For this review, take the finished solid that the model builds, in its own axes (mm). Face numbers are marked on the shaded views. A direction names the side the tool comes from. Round coordinates to 2 decimals unless told otherwise and drop trailing zeros. Loops run counter-clockwise (first coordinate to the right, second up) from the corner with the lowest first, then second, coordinate; pieces in that order, holes last. Notation, with made-up numbers: (80.25, 42.25) -> (105.25, 42.25) arc R23 ccw to (105.25, 69.25) -> close; hole circle Ø2 at (47, -37.5). An arc over 180 degrees is marked (long way). One line per question, with ' | ' between items. Start each with the question number.
1. Consider section D-D (y = -4.75). Write out the cut boundary in (x, z).
2. For pin 1 Ø1 at (x, z) = (-6, 8) entering from +Y; pin 2 Ø3 at (x, z) = (-9.5, 1.5) entering from +Y; pin 3 Ø1 at (y, z) = (1.5, -4.5) entering from +X, all flat-tipped, find the tip position at first contact; note any pin that passes through.
3. Consider section C-C (y = -1.25). Write out the cut boundary in (x, z) (3 decimals), and give its area (3 significant figures).
4. Consider section B-B (z = 16.25). Write out the cut boundary in (x, y).
5. Draft analysis for pull direction X (two halves, no side actions). For the marked faces 4, 5, 6 and 7, state which applies: pulls with the +X half, pulls with the -X half, needs draft (parallel to the pull), parting line crosses it, or undercut.
6. Consider section A-A (x = -9). Write out the cut boundary in (y, z), and give its area (3 significant figures).
7. For the marked faces 1, 2 and 3, list the 3-axis set-ups (+Z, -Z, +X, -X, +Y, -Y) from which the entire face can be reached by the end or side of a thin tool; tool diameter is ignored.
8. Wall thickness on line 1 along Z through (x, y) = (5, -4.75); line 2 along Z through (x, y) = (-9, 0.25); line 3 along Y through (x, z) = (5.75, -17.5): over which ranges is each line inside the solid? List them lowest first.
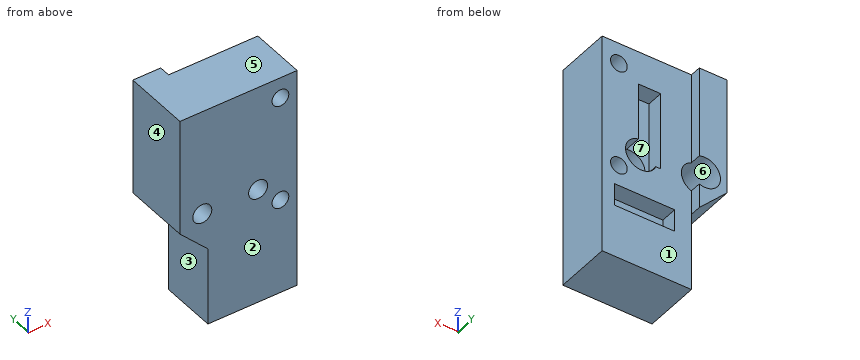
```python
from build123d import *

# Parameters (mm, degrees)
BOX025_W               = 20
BOX025_H               = 10
BOX025_DEPTH           = 44
BOX027_W               = 10.75
BOX027_H               = 10
BOX027_DEPTH           = 4
BOX026_W               = 4
BOX026_H               = 10
BOX026_DEPTH           = 14
CYLINDER031_R          = 2.8
CYLINDER031_DEPTH      = 22
CYLINDER031_ROLL_ANGLE = 90
CYLINDER027_R          = 1.5
CYLINDER027_DEPTH      = 22
CYLINDER027_ROLL_ANGLE = 90
CYLINDER029_R          = 1.5
CYLINDER029_DEPTH      = 22
CYLINDER029_ROLL_ANGLE = 90
CYLINDER026_R          = 1.7
CYLINDER026_DEPTH      = 22
CYLINDER026_ROLL_ANGLE = 90
CYLINDER028_R          = 1.7
CYLINDER028_DEPTH      = 22
CYLINDER028_ROLL_ANGLE = 90
CYLINDER030_R          = 2.8
CYLINDER030_DEPTH      = 22
CYLINDER030_ROLL_ANGLE = 90
PAD016_DEPTH           = 12


with BuildPart() as cube025:
    # Box025 → Box025 (new body)
    with BuildSketch(Plane(origin=(-8, 0, -22), x_dir=(1, 0, 0), z_dir=(0, 0, 1))):
        with Locations((10, 5)):
            Rectangle(BOX025_W, BOX025_H)
    extrude(amount=BOX025_DEPTH)


with BuildPart() as cube027:
    # Box027 → Box027 (new body)
    with BuildSketch(Plane(origin=(-5, -3, -10.5), x_dir=(1, 0, 0), z_dir=(0, 0, 1))):
        with Locations((5.375, 5)):
            Rectangle(BOX027_W, BOX027_H)
    extrude(amount=BOX027_DEPTH)


with BuildPart() as fusion025:
    # Box026 → Box026 (new body)
    with BuildSketch(Plane(origin=(-2.5, -3, 0), x_dir=(1, 0, 0), z_dir=(0, 0, 1))):
        with Locations((2, 5)):
            Rectangle(BOX026_W, BOX026_H)
    extrude(amount=BOX026_DEPTH)

    # Fusion025: union Cube027
    add(cube027.part)


with BuildPart() as cylinder031:
    # Cylinder031 → Cylinder031 (new body)
    with BuildSketch(Plane.XY):
        Circle(CYLINDER031_R)
    extrude(amount=CYLINDER031_DEPTH)


with BuildPart() as cylinder031_1:
    # Cylinder031 roll: moved
    add(cylinder031.part.rotate(Axis((0, 0, 0), (1, 0, 0)), CYLINDER031_ROLL_ANGLE))


with BuildPart() as cylinder031_2:
    # Cylinder031 placement: moved
    add(cylinder031_1.part.moved(Location((-9, 15, 1))))


with BuildPart() as cylinder027:
    # Cylinder027 → Cylinder027 (new body)
    with BuildSketch(Plane.XY):
        Circle(CYLINDER027_R)
    extrude(amount=CYLINDER027_DEPTH)


with BuildPart() as cylinder027_1:
    # Cylinder027 roll: moved
    add(cylinder027.part.rotate(Axis((0, 0, 0), (1, 0, 0)), CYLINDER027_ROLL_ANGLE))


with BuildPart() as cylinder027_2:
    # Cylinder027 placement: moved
    add(cylinder027_1.part.moved(Location((5, 6, 16.25))))


with BuildPart() as cylinder029:
    # Cylinder029 → Cylinder029 (new body)
    with BuildSketch(Plane.XY):
        Circle(CYLINDER029_R)
    extrude(amount=CYLINDER029_DEPTH)


with BuildPart() as cylinder029_1:
    # Cylinder029 roll: moved
    add(cylinder029.part.rotate(Axis((0, 0, 0), (1, 0, 0)), CYLINDER029_ROLL_ANGLE))


with BuildPart() as cylinder029_2:
    # Cylinder029 placement: moved
    add(cylinder029_1.part.moved(Location((5, 6, -2.75))))


with BuildPart() as cylinder026:
    # Cylinder026 → Cylinder026 (new body)
    with BuildSketch(Plane.XY):
        Circle(CYLINDER026_R)
    extrude(amount=CYLINDER026_DEPTH)


with BuildPart() as cylinder026_1:
    # Cylinder026 roll: moved
    add(cylinder026.part.rotate(Axis((0, 0, 0), (1, 0, 0)), CYLINDER026_ROLL_ANGLE))


with BuildPart() as cylinder026_2:
    # Cylinder026 placement: moved
    add(cylinder026_1.part.moved(Location((-9, 6, 1))))


with BuildPart() as cylinder028:
    # Cylinder028 → Cylinder028 (new body)
    with BuildSketch(Plane.XY):
        Circle(CYLINDER028_R)
    extrude(amount=CYLINDER028_DEPTH)


with BuildPart() as cylinder028_1:
    # Cylinder028 roll: moved
    add(cylinder028.part.rotate(Axis((0, 0, 0), (1, 0, 0)), CYLINDER028_ROLL_ANGLE))


with BuildPart() as cylinder028_2:
    # Cylinder028 placement: moved
    add(cylinder028_1.part.moved(Location((1, 6, 1))))


with BuildPart() as fusion024:
    # Cylinder030 → Cylinder030 (new body)
    with BuildSketch(Plane.XY):
        Circle(CYLINDER030_R)
    extrude(amount=CYLINDER030_DEPTH)


with BuildPart() as fusion024_1:
    # Cylinder030 roll: moved
    add(fusion024.part.rotate(Axis((0, 0, 0), (1, 0, 0)), CYLINDER030_ROLL_ANGLE))


with BuildPart() as fusion024_2:
    # Cylinder030 placement: moved
    add(fusion024_1.part.moved(Location((1, 15, 1))))

    # Fusion024: union Cylinder031, Cylinder027, Cylinder029, Cylinder026, Cylinder028
    add(cylinder031_2.part)
    add(cylinder027_2.part)
    add(cylinder029_2.part)
    add(cylinder026_2.part)
    add(cylinder028_2.part)


with BuildPart() as cut036:
    # Sketch018 → Pad016 (new body)
    with BuildSketch(Plane.XZ.offset(-2)):
        Polygon((-13, 20), (8, 20), (8, -20), (-8, -20), (-8, -6), (-13, -1), align=None)
    extrude(amount=PAD016_DEPTH)

    # Cut034: cut Fusion024
    add(fusion024_2.part, mode=Mode.SUBTRACT)

    # Cut035: cut Fusion025
    add(fusion025.part, mode=Mode.SUBTRACT)

    # Cut036: cut Cube025
    add(cube025.part, mode=Mode.SUBTRACT)


solid = cut036.part
```
Answer block:
1) outline: (-13, -1) -> (-8, -6) -> (-8, -20) -> (8, -20) -> (8, 20) -> (-13, 20) -> close; hole circle Ø5.6 at (-9, 1); hole circle Ø5.6 at (1, 1); hole circle Ø3 at (5, -2.75); hole circle Ø3 at (5, 16.25)
2) pin 1: stops at y = 0 | pin 2: stops at y = -7 | pin 3: stops at x = -8
3) outline: (-13, -1) -> (-8, -6) -> (-8, -20) -> (8, -20) -> (8, 20) -> (-13, 20) -> close; hole circle Ø5.6 at (-9, 1); hole (-5, -10.5) -> (5.75, -10.5) -> (5.75, -6.5) -> (-5, -6.5) -> close; hole (-2.5, 0) -> (-1.615, 0) arc R2.8 ccw (long way) to (1.5, 3.755) -> (1.5, 14) -> (-2.5, 14) -> close; hole circle Ø3 at (5, -2.75); hole circle Ø3 at (5, 16.25) | area: 606 mm2
4) outline: (-13, -10) -> (3.5, -10) -> (3.5, 0) -> (-8, 0) -> (-8, 2) -> (-13, 2) -> close; (6.5, -10) -> (8, -10) -> (8, 0) -> (6.5, 0) -> close
5) face 4: pulls with the -X half | face 5: needs draft | face 6: undercut | face 7: undercut
6) outline: (-10, -5) -> (2, -5) -> (2, -1.8) -> (-7, -1.8) -> (-7, -0.7) -> (-10, -0.7) -> close; (-10, 2.7) -> (-7, 2.7) -> (-7, 3.8) -> (2, 3.8) -> (2, 20) -> (-10, 20) -> close | area: 239 mm2
7) face 1: +Z, -Z, +X, +Y | face 2: +Z, -Z, +X, -X, -Y | face 3: -Z, -X, +Y, -Y
8) line 1: z = -20 to -4.25, -1.25 to 14.75, 17.75 to 20 | line 2: z = -5 to -1.8, 3.8 to 20 | line 3: y = -10 to 0
